from build123d import *

# Parameters (mm, degrees)
SKETCH1_W           = 44.45
SKETCH1_H           = 38.1
BOSS_EXTRUDE1_DEPTH = 15.24
SKETCH2_R           = 4.826
BOSS_EXTRUDE2_DEPTH = 3.175
BOSS_EXTRUDE3_DEPTH = 6.35


with BuildPart() as part:
    # Sketch1 → Boss-Extrude1 (new body)
    with BuildSketch(Plane.XY):
        Rectangle(SKETCH1_W, SKETCH1_H)
    extrude(amount=BOSS_EXTRUDE1_DEPTH)

    # Sketch2 → Boss-Extrude2 (add)
    with BuildSketch(Plane(origin=(22.225, 0, 0), x_dir=(0, 0, -1), z_dir=(1, 0, 0))):
        with Locations((-7.62, 6.35)):
            Circle(SKETCH2_R)
    boss_extrude2 = extrude(amount=BOSS_EXTRUDE2_DEPTH)

    # Mirror1: Boss-Extrude2 across plane
    add(boss_extrude2.mirror(Plane(origin=(0, 0, 0), x_dir=(0, 0, 1), z_dir=(1, 0, 0))))

    # Sketch5 → Revolve1 (revolve)
    with BuildSketch(Plane(origin=(0, 0, 0), x_dir=(0, 0, -1), z_dir=(1, 0, 0))):
        with BuildLine():
            Line((-52.07, -19.05), (-7.62, -19.05))
            Line((-7.62, -19.05), (-7.62, -63.5))
            ThreePointArc((-7.62, -63.5), (-39.050896424, -50.480896424), (-52.07, -19.05))
        make_face()
    revolve(axis=Axis((0, -19.05, 7.62), (0, -1, 0)))

    # Sketch7 → Boss-Extrude3 (add, symmetric)
    with BuildSketch(Plane(origin=(0, 0, 0), x_dir=(0, 0, -1), z_dir=(1, 0, 0))):
        Polygon((-15.24, 0), (-15.24, -19.05), (-34.29, -19.05), align=None)
    boss_extrude3 = extrude(amount=BOSS_EXTRUDE3_DEPTH, both=True)

    # Mirror3: Boss-Extrude3 across plane
    add(boss_extrude3.mirror(Plane.XY.offset(7.62)))


solid = part.part
The model under review builds one solid part; all positions refer to its coordinate system, in mm. A direction names the side the tool comes from. Coordinates: 2 decimals unless noted, no trailing zeros. Write each loop counter-clockwise with the first axis right and the second up, starting at its lowest first coordinate (ties: lowest second). Pieces come first, ordered by that corner, then holes. Notation, with made-up numbers: (-12, -4.5) - (11, -4.5) arc R18 ccw to (11, 18.5) - close; hole circle Ø9 at (57, 13). An arc over 180 degrees is marked (long way). Answer as a JSON object with one key per item and string values. Group by question number.
1. To check wall thickness, follow probe 1 along Z at (x, y) = (19, -13.5); probe 2 along X at (y, z) = (-17, 10) (3 decimals); probe 3 along Y at (x, z) = (27.5, 29). State the ranges of each line that lie inside material, in increasing order.
2. Clearance check with flat-ended pins moving along their axes: pin 1 Ø7.5 at (y, z) = (5, 10.5) entering from -X; pin 2 Ø12 at (x, y) = (13.5, -28) entering from -Z; pin 3 Ø5.5 at (y, z) = (-14, 24) entering from +X. State where each tip first meets the part, or that it passes through.
3. Add section D-D (z = -8.5). Give the boundary of the cut face in (x, y), plus the area to 3 significant figures.
4. Add section B-B (z = 7.62). Give the boundary of the cut face in (x, y) (3 decimals), plus the area to 3 significant figures.
5. Machinability: for faces 4 (the face through (6.35, -14, 20)), 5 (the face through (-0.3, 0.3, 0)), 6 (the face through (6.35, -14, -5)), 7 (the face through (-0.3, 0.3, 15.24)), which of the approach directions +Z, -Z, +X, -X, +Y, -Y give a long, thin tool a straight path to every point of the face, cutting with its end or side? Answer none if there is none.
6. Mouldability with a two-part tool opening along Y and no side actions: class faces 1 (the face through (25.4, 6, 8)), 2 (the face through (-22.225, 0, 8)), 3 (the face through (0, 19.05, 8)) as pulls with the +Y half, pulls with the -Y half, needs draft (parallel to the pull), parting line crosses it, or undercut.
7. Add section A-A (y = 6.35). Give the boundary of the cut face in (x, z) (3 decimals), plus the area to 3 significant figures.
8. Add section C-C (x = 12). Give the boundary of the cut face in (y, z).
Findings:
{
 "1": {"probe 1": "0 to 15.24", "probe 2": "-22.225 to 22.225", "probe 3": "-46.66 to -19.05"},
 "2": {"pin 1": "x = -25.4", "pin 2": "z = -35.64", "pin 3": "x = 6.35"},
 "3": {"outline": "(-41.42, -19.05) arc R41.42 ccw to (41.42, -19.05) - (6.35, -19.05) - (6.35, -8.5) - (-6.35, -8.5) - (-6.35, -19.05) - close", "area": "2,830 mm²"},
 "4": {"outline": "(-44.45, -19.05) arc R44.45 ccw to (44.45, -19.05) - (22.225, -19.05) - (22.225, 1.524) - (25.4, 1.524) - (25.4, 11.176) - (22.225, 11.176) - (22.225, 19.05) - (-22.225, 19.05) - (-22.225, 11.176) - (-25.4, 11.176) - (-25.4, 1.524) - (-22.225, 1.524) - (-22.225, -19.05) - close", "area": "4,860 mm²"},
 "5": {"face 4": "+Z, +X, +Y", "face 5": "-Z, +Y", "face 6": "-Z, +X, +Y", "face 7": "+Z, +Y"},
 "6": {"face 1": "needs draft", "face 2": "undercut", "face 3": "pulls with the +Y half"},
 "7": {"outline": "(-25.4, 2.794) - (-22.225, 2.794) - (-22.225, 0) - (22.225, 0) - (22.225, 2.794) - (25.4, 2.794) - (25.4, 12.446) - (22.225, 12.446) - (22.225, 15.24) - (-22.225, 15.24) - (-22.225, 12.446) - (-25.4, 12.446) - close", "area": "739 mm²"},
 "8": {"outline": "(-19.05, -35.18) - (-19.05, 0) - (19.05, 0) - (19.05, 15.24) - (-19.05, 15.24) - (-19.05, 50.42) arc R42.8 ccw to start"}
}
